Design review of the part shown in the three views and the two pictorial views. Dimensions are in mm from the part's minimum x, y and z. A direction names the side the tool comes from. Give positions to 0.01 mm unless a question says otherwise; leave off trailing zeros. Loops run counter-clockwise (first coordinate to the right, second up) from the corner with the lowest first, then second, coordinate; pieces in that order, holes last. Notation, with made-up numbers: (-15.5, -3) - (14.5, -3) arc R35 cw to (14.5, 36) - close; hole circle Ø8 at (-36.5, 28.5). An arc over 180 degrees is marked (long way). Answer in a Markdown table with one row per item.
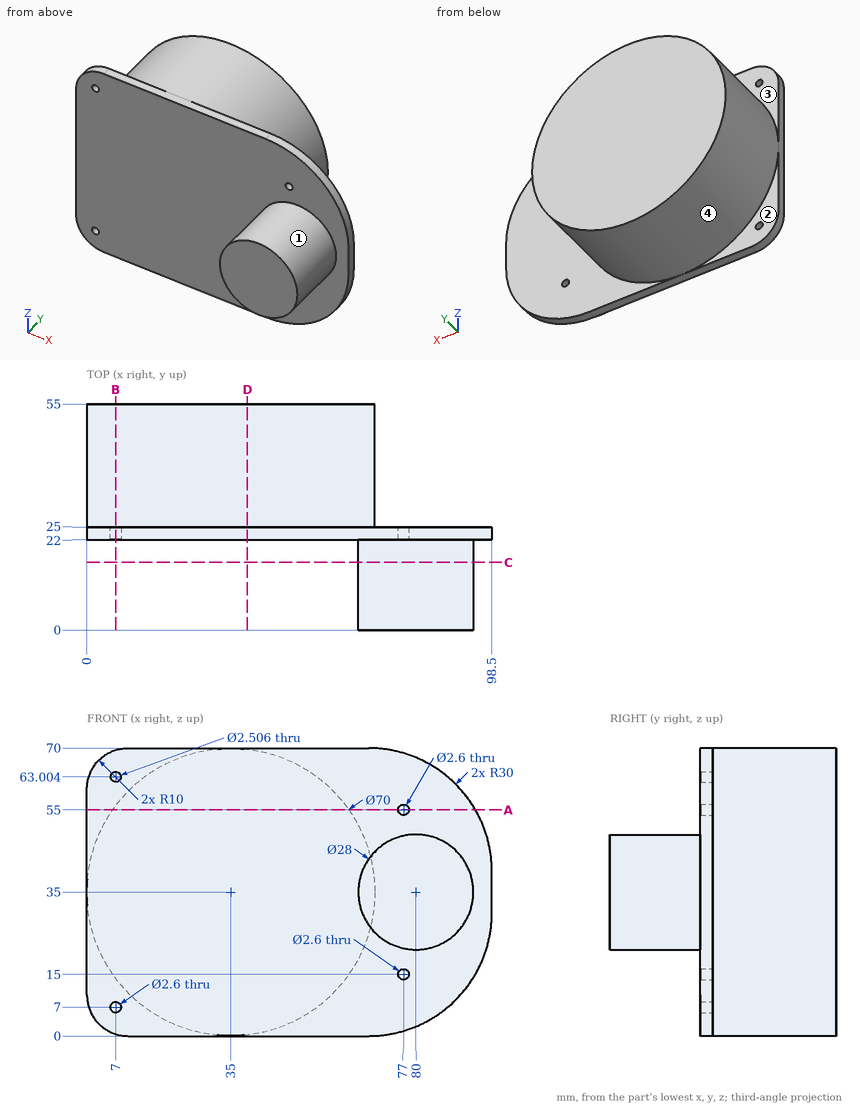
1. We need section D-D, the plane x = 39. Give the boundary of the cut face in (y, z).
Values:
| item | result |
|---|---|
| outline | (22, 0) - (25, 0) - (25, 0.23) - (55, 0.23) - (55, 69.77) - (25, 69.77) - (25, 70) - (22, 70) - close |
2. We need section A-A, the plane z = 55. Give the boundary of the cut face in (x, y).
Values:
| item | result |
|---|---|
| outline | (0, 22) - (75.7, 22) - (75.7, 25) - (63.72, 25) - (63.72, 55) - (6.28, 55) - (6.28, 25) - (0, 25) - close; (78.3, 22) - (94.48, 22) - (94.48, 25) - (78.3, 25) - close |
3. Clearance check with flat-ended pins moving along their axes: pin 1 (5 mm diameter, centred on y = 25, z = 57.5, fed in from +X); pin 2 (4 mm diameter, centred on y = 38.5, z = 29, fed in from +X); pin 3 (3 mm diameter, centred on x = 82, z = 37.5, fed in from +Y). State where each tip first meets the part, or that it passes through.
Values:
| item | result |
|---|---|
| pin 1 | stops at x = 94.48 |
| pin 2 | stops at x = 69.77 |
| pin 3 | stops at y = 25 |
4. For the marked faces 1, 2, 3 and 4, list the 3-axis set-ups (+Z, -Z, +X, -X, +Y, -Y) from which the entire face can be reached by the end or side of a thin tool; tool diameter is ignored.
Values:
| item | result |
|---|---|
| face 1 | -Y |
| face 2 | -Z, -X, +Y |
| face 3 | +Z, -X, +Y |
| face 4 | +Y |
5. We need section B-B, the plane x = 7. Give the boundary of the cut face in (y, z).
Values:
| item | result |
|---|---|
| outline | (22, 0.46) - (25, 0.46) - (25, 5.7) - (22, 5.7) - close; (22, 8.3) - (25, 8.3) - (25, 14) - (55, 14) - (55, 56) - (25, 56) - (25, 61.75) - (22, 61.75) - close; (22, 64.26) - (25, 64.26) - (25, 69.54) - (22, 69.54) - close |
6. We need section C-C, the plane y = 16.5. Give the boundary of the cut face in (x, z), and give its area (3 significant figures).
Values:
| item | result |
|---|---|
| outline | circle Ø28 at (80, 35) |
| area | 616 mm^2 |
7. Wall thickness on line 1 (Z direction, x = 77, y = 23.85); line 2 (Z direction, x = 7, y = 23.65); line 3 (Y direction, x = 41, z = 60): over which ranges is each line inside the solid? List them lowest first. Write a range as [from, to].
Values:
| item | result |
|---|---|
| line 1 | z = [1.23, 13.7], [16.3, 53.7], [56.3, 68.77] |
| line 2 | z = [0.46, 5.7], [8.3, 61.75], [64.26, 69.54] |
| line 3 | y = [22, 55] |
